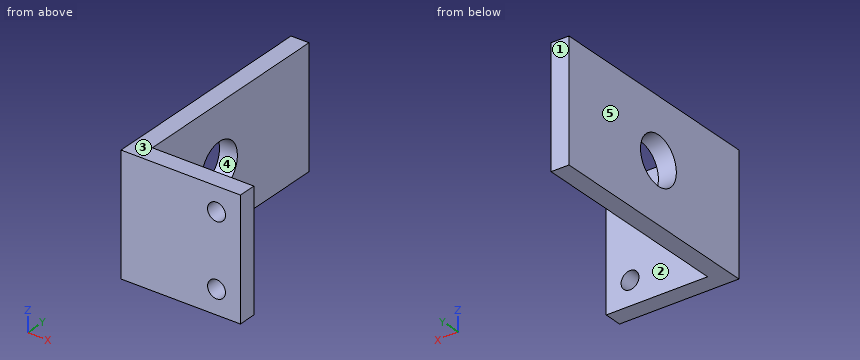
```python
from build123d import *

# Parameters (mm, degrees)
EXTRUDE_1_DEPTH     = 20
SKETCH_2_R          = 1.5
CUT_EXTRUDE_1_DEPTH = 46
SKETCH_3_R          = 4
CUT_EXTRUDE_2_DEPTH = 47.184412955


with BuildPart() as part:
    # 草图1 → 凸台-拉伸1 (new body)
    with BuildSketch(Plane.XY):
        Polygon((0, 0), (0, 38), (3, 38), (3, 3), (20, 3), (20, 0), align=None)
    extrude(amount=EXTRUDE_1_DEPTH)

    # 草图2 → 切除-拉伸1 (cut, through all)
    with BuildSketch(Plane(origin=(0, 3, 0), x_dir=(1, 0, 0), z_dir=(0, 1, 0))):
        with Locations(Location((16, -16, 0), (0, 0, 270))):
            Circle(SKETCH_2_R)
        with Locations(Location((16, -4, 0), (0, 0, 270))):
            Circle(SKETCH_2_R)
    extrude(amount=-CUT_EXTRUDE_1_DEPTH, mode=Mode.SUBTRACT)

    # 草图3 → 切除-拉伸2 (cut, through all)
    with BuildSketch(Plane(origin=(3, 0, 0), x_dir=(0, 0, -1), z_dir=(1, 0, 0))):
        with Locations(Location((-10, 18, 0), (0, 0, 90))):
            Circle(SKETCH_3_R)
    extrude(amount=-CUT_EXTRUDE_2_DEPTH, mode=Mode.SUBTRACT)


solid = part.part
```
Verification items for the finished model (mm, model axes). Face numbers are marked on the shaded views. A direction names the side the tool comes from. Round coordinates to 2 decimals unless told otherwise and drop trailing zeros. Write each loop counter-clockwise with the first axis right and the second up, starting at its lowest first coordinate (ties: lowest second). Pieces come first, ordered by that corner, then holes. Notation, with made-up numbers: (42.5, 4) - (100.5, 4) arc R7 cw to (100.5, 17) - close; hole circle Ø11 at (-39.5, 12). An arc over 180 degrees is marked (long way). Answer as a JSON object with one key per item and string values. Group by question number.
Q1. Section check B-B, the plane z = 10. Enter the section's corners in (x, y), plus the area to 3 significant figures.
Q2. Go/stop test with flat-tipped pins: pin 1 Ø1 at (y, z) = (12, 15.5) entering from +X; pin 2 Ø4 at (x, z) = (16, 16) entering from +Y. Record where each tip stops, or that it passes through.
Q3. Thickness scan on line 1 (Z direction, x = 1.05, y = 18); line 2 (X direction, y = 34, z = 16.5). Record the ranges inside material, lowest first.
Q4. Section check A-A, the plane y = 18. Enter the section's corners in (x, z).
Q5. Section check C-C, the plane x = 16. Enter the section's corners in (y, z), plus the area to 3 significant figures.
Q6. Tool access check on the marked faces 1 and 2. Record the directions out of +Z, -Z, +X, -X, +Y, -Y that give a thin tool (end or side, any length) a straight path to the whole face; none if there is none.
Q7. Mould release check, pull along Z, two halves, no side actions. Record for the marked faces 3, 4 and 5: released by +Z, released by -Z, zero draft, split by the parting line, or undercut.
Q8. Section check D-D, the plane z = 2. Enter the section's corners in (x, y).
Found:
{
 "1": {"outline": "(0, 0) - (20, 0) - (20, 3) - (3, 3) - (3, 14) - (0, 14) - close; (0, 22) - (3, 22) - (3, 38) - (0, 38) - close", "area": "141 mm^2"},
 "2": {"pin 1": "stops at x = 3", "pin 2": "stops at y = 3"},
 "3": {"line 1": "z = 0 to 6, 14 to 20", "line 2": "x = 0 to 3"},
 "4": {"outline": "(0, 0) - (3, 0) - (3, 6) - (0, 6) - close; (0, 14) - (3, 14) - (3, 20) - (0, 20) - close"},
 "5": {"outline": "(0, 0) - (3, 0) - (3, 2.5) - (0, 2.5) - close; (0, 5.5) - (3, 5.5) - (3, 14.5) - (0, 14.5) - close; (0, 17.5) - (3, 17.5) - (3, 20) - (0, 20) - close", "area": "42.0 mm^2"},
 "6": {"face 1": "+Z, -Z, +X, -X, +Y", "face 2": "+Z, -Z, +X, +Y"},
 "7": {"face 3": "released by +Z", "face 4": "undercut", "face 5": "zero draft"},
 "8": {"outline": "(0, 0) - (20, 0) - (20, 3) - (3, 3) - (3, 38) - (0, 38) - close"}
}
